```python
from build123d import *

# Parameters (mm, degrees)
F1_DEPTH = 908.05
F2_R     = 1.27
F3_R     = 3.175


with BuildPart() as f1:
    # F0 (on Top) → F1 (new body)
    with BuildSketch(Plane.XY):
        with BuildLine():
            ThreePointArc((49.2125, -11.1125), (51.457564, -10.182564), (52.3875, -7.9375))
            Line((52.3875, -7.9375), (46.0375, -7.9375))
            ThreePointArc((46.0375, -7.9375), (46.967436, -10.182564), (49.2125, -11.1125))
        make_face()
        with BuildLine():
            ThreePointArc((42.8625, -11.1125), (45.107564, -10.182564), (46.0375, -7.9375))
            Line((46.0375, -7.9375), (39.6875, -7.9375))
            ThreePointArc((39.6875, -7.9375), (40.617436, -10.182564), (42.8625, -11.1125))
        make_face()
        with BuildLine():
            ThreePointArc((36.5125, -11.1125), (38.757564, -10.182564), (39.6875, -7.9375))
            Line((39.6875, -7.9375), (33.3375, -7.9375))
            ThreePointArc((33.3375, -7.9375), (34.267436, -10.182564), (36.5125, -11.1125))
        make_face()
        Polygon((52.3875, 3.704167), (52.3875, 11.1125), (-58.7375, 11.1125), (-58.7375, 3.704167), (-52.3875, 3.704167), (-52.3875, -3.704167), (-58.7375, -3.704167), (-58.7375, -11.1125), (33.3375, -11.1125), (33.3375, -7.9375), (39.6875, -7.9375), (46.0375, -7.9375), (52.3875, -7.9375), (52.3875, -3.704167), (58.7375, -3.704167), (58.7375, 3.704167), align=None)
    extrude(amount=F1_DEPTH)

    # F2
    f2_edges = [f1.edges().sort_by_distance(p)[0] for p in [
        (33.3375, -11.1125, 454.025),
    ]]
    fillet(f2_edges, radius=F2_R)

    # F3
    f3_edges = [f1.edges().sort_by_distance(p)[0] for p in [
        (58.7375, -3.704167, 454.025),
        (58.7375, 3.704167, 454.025),
    ]]
    fillet(f3_edges, radius=F3_R)


solid = f1.part
```
Design review of the part built by this model. Coordinates are the model's own, in mm. Coordinates: 2 decimals unless noted, no trailing zeros. Loops run counter-clockwise (first coordinate to the right, second up) from the corner with the lowest first, then second, coordinate; pieces in that order, holes last. Notation, with made-up numbers: (63.5, 9.25) - (94.5, 9.25) arc R16 cw to (94.5, 40.25) - close; hole circle Ø3 at (66.25, 88.25). An arc over 180 degrees is marked (long way). Use CSV: the item, a comma, the result in double quotes. Start each with the question number.
1) For pin 1 Ø3.5 at (x, z) = (54, 572.5) entering from +Y; pin 2 Ø1 at (y, z) = (-9.5, 299) entering from +X; pin 3 Ø1 at (x, z) = (54.5, 561) entering from -Y; pin 4 Ø2 at (y, z) = (-6.5, 354) entering from +X, all flat-tipped, find the tip position at first contact; note any pin that passes through.
2) Consider section B-B on y = 7.5. Write out the cut boundary in (x, z).
3) Wall thickness on L1, parallel to X at y = -1, z = 164.5; L2, parallel to Y at x = 39, z = 279; L3, parallel to X at y = 10.25, z = 670: over which ranges is each line inside the solid? List them lowest first. Write a range as from..to.
Geometry says:
1,pin 1,"y = 11.11"
1,pin 2,"x = 52.2"
1,pin 3,"y = -3.7"
1,pin 4,"x = 52.39"
2,outline,"(-58.74, 0) - (52.39, 0) - (52.39, 908.05) - (-58.74, 908.05) - close"
3,L1,"-52.39..58.7"
3,L2,"-9.91..11.11"
3,L3,"-58.74..52.39"
